from build123d import *

# Parameters (mm, degrees)
BOSS_EXTRUDE1_DEPTH = 38.1
SKETCH3_R           = 14.2875
SKETCH3_R_2         = 1.7272
CUT_EXTRUDE1_DEPTH  = 61.658289829
SKETCH9_R           = 2.4892
CUT_EXTRUDE2_DEPTH  = 77.464125575


with BuildPart() as part:
    # Sketch2 → Boss-Extrude1 (new, symmetric)
    with BuildSketch(Plane.XY):
        with BuildLine():
            Line((-19.05, -31.75), (19.05, -31.75))
            Line((19.05, -31.75), (19.05, 31.75))
            Line((19.05, 31.75), (17.4625, 31.75))
            ThreePointArc((17.4625, 31.75), (16.339967985, 31.285032015), (15.875, 30.1625))
            Line((15.875, 30.1625), (15.875, -23.7998))
            ThreePointArc((15.875, -23.7998), (14.476376302, -27.176376302), (11.0998, -28.575))
            Line((11.0998, -28.575), (-17.4625, -28.575))
            ThreePointArc((-17.4625, -28.575), (-18.585032015, -29.039967985), (-19.05, -30.1625))
            Line((-19.05, -30.1625), (-19.05, -31.75))
        make_face()
    extrude(amount=BOSS_EXTRUDE1_DEPTH, both=True)

    # Sketch3 → Cut-Extrude1 (cut, through all)
    with BuildSketch(Plane.ZY.offset(-15.875)):
        with Locations(Location((12.70000005, 3.1797625, 0), (0, 0, 270))):
            Circle(SKETCH3_R)
        with Locations(Location((25.451963742, 15.931726192, 0), (0, 0, 270))):
            Circle(SKETCH3_R_2)
    extrude(amount=-CUT_EXTRUDE1_DEPTH, mode=Mode.SUBTRACT)

    # Sketch9 → Cut-Extrude2 (cut, through all)
    with BuildSketch(Plane.XZ.offset(31.75)):
        Circle(SKETCH9_R)
        with Locations((0, -25.4)):
            Circle(SKETCH9_R)
    extrude(amount=-CUT_EXTRUDE2_DEPTH, mode=Mode.SUBTRACT)


solid = part.part
Can you work these out from the model? Positions are in its coordinate system, mm. A direction names the side the tool comes from. Round coordinates to 2 decimals unless told otherwise and drop trailing zeros. Write each loop counter-clockwise with the first axis right and the second up, starting at its lowest first coordinate (ties: lowest second). Pieces come first, ordered by that corner, then holes. Notation, with made-up numbers: (0.5, 73.5) -> (41.5, 73.5) arc R25 cw to (41.5, 87.5) -> close; hole circle Ø6 at (-14.75, 61). An arc over 180 degrees is marked (long way). Use one line per item in the form item = value. Start each with the question number.
Q1. If I drill on probe 1 along Z at (x, y) = (0, -29); probe 2 along Y at (x, z) = (10, 6.5) (3 decimals); probe 3 along X at (y, z) = (15.5, 27.5) (3 decimals), over which ranges is the centre line in solid material (lowest first)? Write a range as [from, to].
Q2. Imagine slicing it at D-D (z = 0). Count the separate pieces of the cut face and the enclosed holes in it, then the cut area to 3 significant figures.
Q3. I'm going to push flat-ended pins straight in: P1, Ø8, axis at x = 8.5, z = 8, coming from the +Y side; P2, Ø8.5, axis at x = -3, z = 1.5, coming from the +Y side (3 decimals); P3, Ø23, axis at y = 3.18, z = 12.7, coming from the +X side; P4, Ø1.5, axis at y = 16.5, z = 21, coming from the -X side (3 decimals). Where does each tip first touch, or does it pass through?
Q4. Imagine slicing it at A-A (x = 0). Please give me the cut outline in (y, z) (3 decimals), then the cut area to 3 significant figures.
Q5. Which directions (+Z, -Z, +X, -X, +Y, -Y) give clear straight access to the entire face, cutting with the end or side of a thin tool? Please do faces 4 (the face through (-3, -28.575, 1)), 5 (the face through (2.374, -30.185, 0.748)).
Q6. We'd pull the mould along X, two halves only. Please class faces 1 (the face through (19.05, 0, -8)), 2 (the face through (-0.54, -30.18, -27.83)), 3 (the face through (15.875, 4, -8)): +X half, -X half, draft (parallel to the pull), parting line (faces both ways), or undercut.
Q7. Imagine slicing it at C-C (y = -3). Please give me the cut outline in (x, z) (3 decimals).
Worked out:
q1.probe_1 = [-38.1, -27.89], [-22.91, -2.49], [2.49, 38.1]
q1.probe_2 = [-31.75, -28.575]
q1.probe_3 = [15.875, 19.05]
q2.separate_pieces = 3
q2.enclosed_holes = 0
q2.area = 259 mm^2
q3.P1 = -28.37
q3.P2 = -28.575
q3.P3 = through
q3.P4 = 15.875
q4.outline = (-31.75, -38.1) -> (-28.575, -38.1) -> (-28.575, -27.889) -> (-31.75, -27.889) -> close; (-31.75, -22.911) -> (-28.575, -22.911) -> (-28.575, -2.489) -> (-31.75, -2.489) -> close; (-31.75, 2.489) -> (-28.575, 2.489) -> (-28.575, 38.1) -> (-31.75, 38.1) -> close
q4.area = 210 mm^2
q5.face_4 = +Z, -Z, -X, +Y
q5.face_5 = +Y, -Y
q6.face_1 = +X half
q6.face_2 = undercut
q6.face_3 = -X half
q7.outline = (15.875, -38.1) -> (19.05, -38.1) -> (19.05, -0.182) -> (15.875, -0.182) -> close; (15.875, 25.582) -> (19.05, 25.582) -> (19.05, 38.1) -> (15.875, 38.1) -> close
